from build123d import *

# Parameters (mm, degrees)
F0_R     = 3.175
F1_DEPTH = 6.35


with BuildPart() as f1:
    # F0 (on Right) → F1 (new body)
    with BuildSketch(Plane.YZ):
        with BuildLine():
            Line((58.42, 6.35), (0, 6.35))
            ThreePointArc((0, 6.35), (-6.35, 0), (0, -6.35))
            Line((0, -6.35), (58.42, -6.35))
            ThreePointArc((58.42, -6.35), (64.77, 0), (58.42, 6.35))
        make_face()
        Circle(F0_R, mode=Mode.SUBTRACT)
        with Locations((58.42, 0)):
            Circle(F0_R, mode=Mode.SUBTRACT)
    extrude(amount=F1_DEPTH)


solid = f1.part
Geometry: final body of the model. Coordinates: model frame, mm. Give positions to 0.01 mm unless a question says otherwise; leave off trailing zeros. Order: outer loops, then holes, each group sorted by start corner. A loop starts at its lowest first (then second) coordinate and runs counter-clockwise, first axis right, second up. Notation, with made-up numbers: (84, 64.25) -> (109, 64.25) arc R27 cw to (109, 89.25) -> close; hole circle Ø4 at (-9, -6.5). An arc over 180 degrees is marked (long way). Answer as a JSON object with one key per item and string values.
Q1. Section C-C (z = 5.5). Output: boundary loops of the cut face in (x, y), plus the area to 3 significant figures.
Entries:
{"outline": "(0, -3.17) -> (6.35, -3.17) -> (6.35, 61.59) -> (0, 61.59) -> close", "area": "411 mm^2"}
Q2. Section B-B (x = 3.5). Output: boundary loops of the cut face in (y, z) (3 decimals).
Entries:
{"outline": "(0, -6.35) -> (58.42, -6.35) arc R6.35 ccw to (58.42, 6.35) -> (0, 6.35) arc R6.35 ccw to start; hole circle Ø6.35 at (0, 0); hole circle Ø6.35 at (58.42, 0)"}
Q3. First-contact query: pin 1 (2 mm diameter, centred on x = 4, z = -3.5, fed in from -Y). Flat tip, straight axial feed; report the tip coordinate or a pass-through.
Entries:
{"pin 1": "stops at y = -5.84"}
Q4. Draft query along Y for faces 1 (the cylindrical face through (3.13, -6.35, 0.14)), 2 (the cylindrical face through (3.13, -0.69, -3.1)), 3 (the cylindrical face through (3.13, 64.77, -0.14)). Return one class per face: released by +Y, released by -Y, zero draft, split by the parting line, or undercut.
Entries:
{"face 1": "released by -Y", "face 2": "undercut", "face 3": "released by +Y"}
Q5. Section D-D (z = -4). Output: boundary loops of the cut face in (x, y).
Entries:
{"outline": "(0, -4.93) -> (6.35, -4.93) -> (6.35, 63.35) -> (0, 63.35) -> close"}
Q6. Section A-A (z = 0). Output: boundary loops of the cut face in (x, y) (3 decimals), plus the area to 3 significant figures.
Entries:
{"outline": "(0, -6.35) -> (6.35, -6.35) -> (6.35, -3.175) -> (0, -3.175) -> close; (0, 3.175) -> (6.35, 3.175) -> (6.35, 55.245) -> (0, 55.245) -> close; (0, 61.595) -> (6.35, 61.595) -> (6.35, 64.77) -> (0, 64.77) -> close", "area": "371 mm^2"}
Q7. Material intervals for probe 1 along Z at (x, y) = (5.25, 0) (3 decimals); probe 2 along Y at (x, z) = (6, 1.75); probe 3 along Y at (x, z) = (1, 1), sorted ascending.
Entries:
{"probe 1": "z = -6.35 to -3.175, 3.175 to 6.35", "probe 2": "y = -6.1 to -2.65, 2.65 to 55.77, 61.07 to 64.52", "probe 3": "y = -6.27 to -3.01, 3.01 to 55.41, 61.43 to 64.69"}
